Autodesk Fusion 360 part; units mm, degrees
sketch "Colour Detection Mechanism Platform" plane through (0, 0, 0) normal (0, 0, 1) x (1, 0, 0)
  line L0 (0, 0) -> (120, 0)
  line L1 (120, 0) -> (120, 76)
  line L2 (120, 76) -> (0, 76)
  line L3 (0, 76) -> (0, 0)
  dimension "d169" = 120
  dimension "d170" = 76
extrude "Extrude42" add sketch "Colour Detection Mechanism Platform" along normal blind 4
sketch "Smartie Path" plane through (0, 0, 4) normal (0, 0, 1) x (-1, 0, 0)
  line L0 (0, -76) -> (0, 0)
  line L1 (0, 0) -> (-120, 0)
  line L2 (-120, 0) -> (-120, -76)
  line L3 (-120, -76) -> (0, -76)
  circle A0 centre (-98.5, 24) radius 80
  line L4 (-98.5, 24) -> (-113.5, 24)
  line L5 (-113.5, 24) -> (-113.5, -56)
  line L6 (-113.5, -56) -> (-98.5, -56)
  line L7 (-98.5, -56) -> (-98.5, 24)
  line L8 (-98.5, 24) -> (-18.5, 24)
  line L9 (-18.5, 24) -> (-18.5, 39)
  line L10 (-18.5, 39) -> (-98.5, 39)
  line L11 (-98.5, 39) -> (-98.5, 24)
  line L12 (-98.5, 24) -> (-113.5, 24)
  line L13 (-113.5, 24) -> (-113.5, 39)
  line L14 (-113.5, 39) -> (-98.5, 39)
  line L15 (-98.5, 39) -> (-98.5, 24)
  circle A1 centre (-32.5, 24) radius 9
  dimension "d173" = 160
  dimension "d174" = 24
  dimension "d175" = 21.5
  dimension "d176" = 15
  dimension "d177" = 15
  dimension "d178" = 80
  dimension "d179" = 80
  dimension "d184" = 18
  dimension "d185" = 14
extrude "Extrude43" add sketch "Smartie Path" along normal blind 2 contours L1 A0 L7 | L1 A0 L7 L8 A1 | L1 A0 L5 L7 | L1 L4 L5 L7 L12 | A0 L8 L10 L11 L15 A1 | L4 L11 L12 L13 L14 L15
fillet "Fillet2" radius 15 2 edges at (19.9188, -39, 5) (113.5, 54.5812, 5)
extrude "Extrude44" add 1 faces at (89.4665, -20.5529, 4) along direction (0, 0, -1) blind 4
sketch "Servo Hole" plane through (0, 0, 6) normal (0, 0, 1) x (-1, 0, 0)
  circle A0 centre (-32.5, 24) radius 9
  arc A1 (-113.5, -41) -> (-98.5, -56) centre (-98.5, -41) ccw
  arc A2 (-98.5, -56) -> (-18.5, 24) centre (-98.5, 24) ccw
  arc A3 (-18.5, 24) -> (-33.5, 39) centre (-33.5, 24) ccw
  line L0 (-33.5, 39) -> (-113.5, 39)
  line L1 (-113.5, 39) -> (-113.5, -41)
  line L2 (-113.5, 39) -> (-83.5, 39)
  line L3 (-83.5, 39) -> (-83.5, 9)
  line L4 (-83.5, 9) -> (-113.5, 9)
  line L5 (-113.5, 9) -> (-113.5, 39)
  dimension "d188" = 30
  dimension "d189" = 30
extrude "Extrude45" cut sketch "Servo Hole" against normal blind 6 contours L0 L1 L2 L3 L4 L5
sketch "Colour Sensor Holder Hole" plane through (0, 0, 4) normal (0, 0, 1) x (-1, 0, 0)
  line L0 (-120, 0) -> (-120, -76)
  line L1 (-120, -76) -> (0, -76)
  line L2 (0, -76) -> (0, 0)
  line L3 (-113.5, 0) -> (-120, 0)
  arc A0 (-98.5, -56) -> (-22.1849, 0) centre (-98.5, 24) ccw
  arc A1 (-113.5, -41) -> (-98.5, -56) centre (-98.5, -41) ccw
  line L4 (-113.5, -41) -> (-113.5, 0)
  line L5 (0, -59.401) -> (-38.732, -33.6675)
  line L6 (0, -23.4021) -> (-22.139, -8.693)
  line L7 (-38.732, -33.6675) -> (-22.139, -8.693)
  line L8 (0, -60.0013) -> (-39.4252, -33.8073)
  line L9 (-39.4252, -33.8073) -> (-22.2788, -7.9998)
  line L10 (-22.2788, -7.9998) -> (0, -22.8018)
  line L11 (0, 0) -> (-22.1849, 0)
  dimension "d249" = 56.4
  dimension "d250" = 59.401
  dimension "d254" = 56.4
  dimension "d255" = 8.693
  dimension "d256" = 22.139
  dimension "d257" = 23.4021
  dimension "d258" = 38.732
  dimension "d261" = 0.5
  dimension "d262" = 0.5
  dimension "d263" = 0.5
extrude "Extrude58" cut sketch "Colour Sensor Holder Hole" against normal blind 4 contours L2 L5 L6 L7
extrude "Extrude59" cut sketch "Colour Sensor Holder Hole" against normal blind 4 contours L2 L5 L6 L7 L8 L9 L10
sketch "Platform Extension" plane through (0, 0, 4) normal (0, 0, 1) x (-1, 0, 0)
  line L0 (-22.2788, -7.9998) -> (0, -22.8018)
  line L1 (0, -22.8018) -> (0, 0)
  line L2 (0, 0) -> (-22.1849, 0)
  arc A0 (-98.5, -56) -> (-22.1849, 0) centre (-98.5, 24) ccw
  arc A1 (-113.5, -41) -> (-98.5, -56) centre (-98.5, -41) ccw
  line L3 (-113.5, -41) -> (-113.5, 0)
  line L4 (-120, 0) -> (-120, -76)
  line L5 (-120, -76) -> (0, -76)
  line L6 (0, -60.0013) -> (-39.4252, -33.8073)
  line L7 (-39.4252, -33.8073) -> (-22.2788, -7.9998)
  line L8 (-83.5, 9) -> (-113.5, 9)
  line L9 (-113.5, 9) -> (-113.5, -41)
  arc A2 (-113.5, -41) -> (-98.5, -56) centre (-98.5, -41) ccw
  arc A3 (-98.5, -56) -> (-18.5, 24) centre (-98.5, 24) ccw
  arc A4 (-18.5, 24) -> (-33.5, 39) centre (-33.5, 24) ccw
  line L10 (-33.5, 39) -> (-83.5, 39)
  line L11 (-83.5, 39) -> (-83.5, 9)
  circle A5 centre (-32.5, 24) radius 9
  line L12 (0, 0) -> (0, 39)
  line L13 (0, 39) -> (-33.5, 39)
  line L14 (-113.5, 0) -> (-120, 0)
  line L15 (0, -76) -> (0, -60.0013)
  line L16 (-113.5, 0) -> (-120, 0)
  line L17 (-120, 0) -> (-120, 9)
  line L18 (-120, 9) -> (-113.5, 9)
  line L19 (-113.5, 9) -> (-113.5, 0)
extrude "Extrude60" add sketch "Platform Extension" against normal blind 4 contours L2 A3 A4 L12 L13 | L9 L14 L16 L17 L18 L19
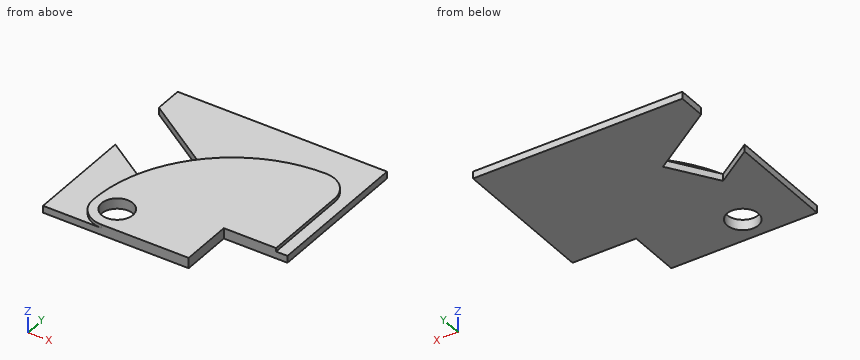
Check sheet for the modelled part. Datum: model origin and axes. Units: mm. Give positions to 0.01 mm unless a question says otherwise; leave off trailing zeros. Loops run counter-clockwise (first coordinate to the right, second up) from the corner with the lowest first, then second, coordinate; pieces in that order, holes last. Notation, with made-up numbers: M -28,64.5 L -20,64.5 A26 cw -20,94.5 Z; hole C 68,22.25 d2. An arc over 180 degrees is marked long. Answer in a Markdown table with one row per item.
1) Cross-section at C-C (x = 29). Enter the section's corners in (y, z).
Solutions:
| item | result |
|---|---|
| outline | M -39,0 L -32.29,0 L -32.29,6 L -38.31,6 L -38.31,4 L -39,4 Z; M -15.71,0 L 18.12,0 L 18.12,4 L 15.62,4 L 15.62,6 L -15.71,6 Z; M 40.73,0 L 76,0 L 76,4 L 40.73,4 Z |
2) Cross-section at D-D (y = 39). Enter the section's corners in (x, z), plus the area to 3 significant figures.
Solutions:
| item | result |
|---|---|
| outline | M 31.61,0 L 120,0 L 120,4 L 113.5,4 L 113.5,6 L 49.19,6 L 49.19,4 L 31.61,4 Z |
| area | 482 mm^2 |
3) Depth check by flat-ended pin: pin 1 (1.5 mm diameter, centred on y = 25, z = 2.5, fed in from -X); pin 2 (3 mm diameter, centred on x = 93.5, z = 1, fed in from -Y); pin 3 (1.6 mm diameter, centred on y = 19.5, z = 5.5, fed in from +X); pin 4 (11 mm diameter, centred on x = 32.5, y = -24, fed in from +Z). Enter the tip coordinate at first touch or a pass-through.
Solutions:
| item | result |
|---|---|
| pin 1 | stops at x = 33.08 |
| pin 2 | stops at y = -9 |
| pin 3 | stops at x = 113.5 |
| pin 4 | passes through |
4) Cross-section at A-A (z = 1.3). Enter the section's corners in (x, y), plus the area to 3 significant figures.
Solutions:
| item | result |
|---|---|
| outline | M 0,-39 L 83.5,-39 L 83.5,-9 L 120,-9 L 120,76 L 0,76 L 0,60 L 39.43,33.81 L 22.28,8 L 0,22.8 Z; hole C 32.5,-24 d18 |
| area | 11,300 mm^2 |
5) Thickness scan on line 1 (X direction, y = -24, z = 4.35); line 2 (X direction, y = -24, z = 3.3); line 3 (Z direction, x = 5.5, y = -32). Record the ranges inside material, lowest first.
Solutions:
| item | result |
|---|---|
| line 1 | x = 18.5 to 23.5, 41.5 to 83.5 |
| line 2 | x = 0 to 23.5, 41.5 to 83.5 |
| line 3 | z = 0 to 4 |
6) Cross-section at B-B (y = 16.5). Enter the section's corners in (x, z), plus the area to 3 significant figures.
Solutions:
| item | result |
|---|---|
| outline | M 0,0 L 9.48,0 L 9.48,4 L 0,4 Z; M 27.93,0 L 120,0 L 120,4 L 113.5,4 L 113.5,6 L 29.51,6 L 29.51,4 L 27.93,4 Z |
| area | 574 mm^2 |
